Design review of the part shown in the three views and the two pictorial views. Dimensions are in mm from the part's minimum x, y and z. Round coordinates to 2 decimals unless told otherwise and drop trailing zeros. Order: outer loops, then holes, each group sorted by start corner. A loop starts at its lowest first (then second) coordinate and runs counter-clockwise, first axis right, second up. Notation, with made-up numbers: (62.25, -26.5) - (88.25, -26.5) arc R9 cw to (88.25, -12.5) - close; hole circle Ø5 at (17.5, 76). An arc over 180 degrees is marked (long way). One line per item, written item: value.
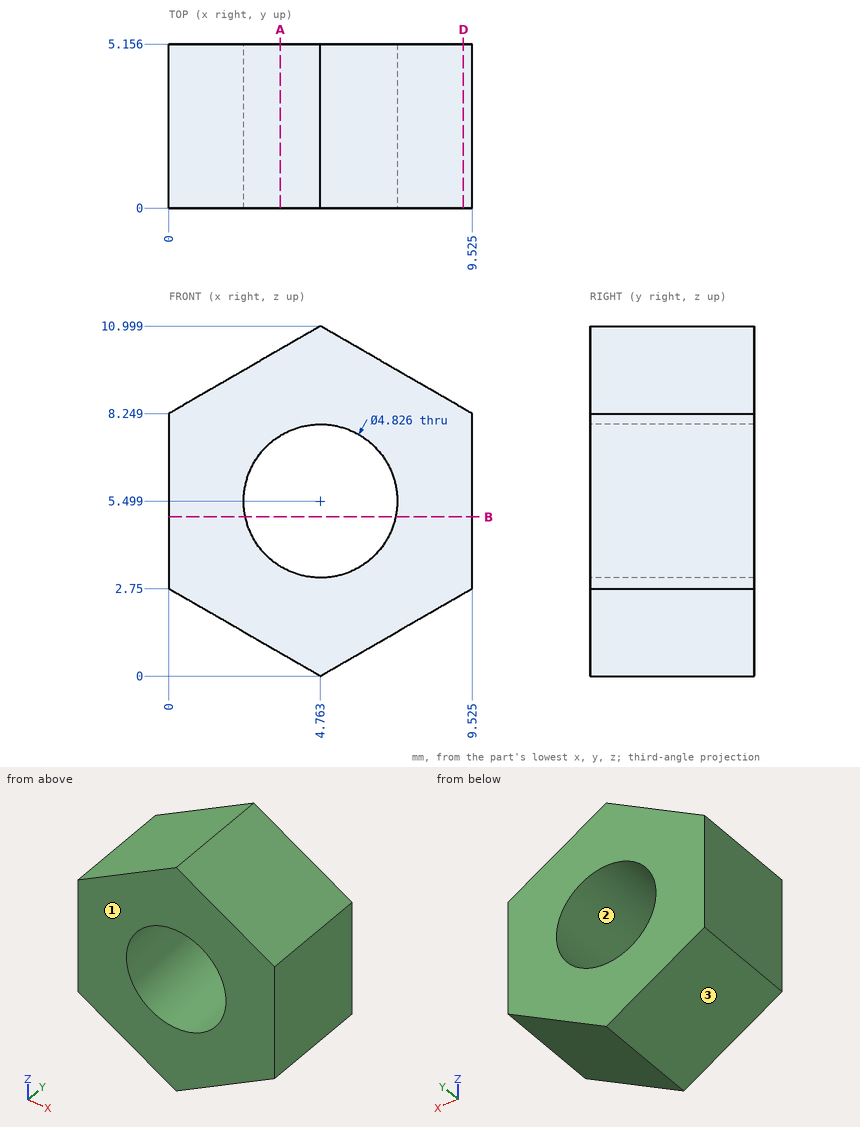
Item 1: The part is to be moulded in two halves that separate along X. For the marked faces 1, 2 and 3, say which applies: +X half, -X half, draft (parallel to the pull), parting line (faces both ways), or undercut.
Returned:
face 1: draft
face 2: undercut
face 3: -X half
Item 2: Wall thickness on line 1 (X direction, y = 1.3, z = 3.5) (1 decimal); line 2 (Z direction, x = 6.25, y = 2.8); line 3 (X direction, y = 3.15, z = 4.75) (1 decimal): over which ranges is each line inside the solid? List them lowest first.
Returned:
line 1: 0 to 3.4, 6.1 to 9.5
line 2: 0.86 to 3.6, 7.4 to 10.14
line 3: 0 to 2.5, 7.1 to 9.5
Item 3: Take a section at D-D (x = 9.25). Write out the cut boundary in (y, z), plus the area to 3 significant figures.
Returned:
outline: (0, 2.59) - (5.16, 2.59) - (5.16, 8.41) - (0, 8.41) - close
area: 30.0 mm^2
Item 4: Take a section at A-A (x = 3.5). Write out the cut boundary in (y, z) (1 decimal), plus the area to 3 significant figures.
Returned:
outline: (0, 0.7) - (5.2, 0.7) - (5.2, 3.4) - (0, 3.4) - close; (0, 7.6) - (5.2, 7.6) - (5.2, 10.3) - (0, 10.3) - close
area: 28.0 mm^2
Item 5: Take a section at B-B (z = 5). Write out the cut boundary in (x, y) (1 decimal).
Returned:
outline: (0, 0) - (2.4, 0) - (2.4, 5.2) - (0, 5.2) - close; (7.1, 0) - (9.5, 0) - (9.5, 5.2) - (7.1, 5.2) - close
